Answer from the drawing. Dimensions are ordinates in mm from the lowest x, y and z of the part. A direction names the side the tool comes from. Round coordinates to 2 decimals unless told otherwise and drop trailing zeros. Loops run counter-clockwise (first coordinate to the right, second up) from the corner with the lowest first, then second, coordinate; pieces in that order, holes last. Notation, with made-up numbers: (75.25, -32) - (97.25, -32) arc R21 ccw to (97.25, -12) - close; hole circle Ø11 at (89, 28). An arc over 180 degrees is marked (long way). Answer as CSV lines item,"result". Start each with the question number.
Q1. Section B-B on x = 8 is taken. Write down the section's boundary in (y, z).
Q2. Section C-C on y = 36 is taken. Write down the section's boundary in (x, z), then the cut area to 3 significant figures.
Q3. For the marked faces 4, 5 and 6, determine the directions among +Z, -Z, +X, -X, +Y, -Y from which every point of the face is accessible in a straight line to the end or side of a thin tool.
Q4. Each of these flat-tipped pins is pushed along its axis until it touches: pin 1 Ø11 at (x, z) = (10, 34.5) entering from +Y; pin 2 Ø8 at (y, z) = (36, 25) entering from -X; pin 3 Ø12 at (y, z) = (28, 21) entering from -X; pin 4 Ø12 at (y, z) = (33.5, 30) entering from +X. Where does it stop, or does it pass through?
Q5. Section A-A on y = 30 is taken. Write down the section's boundary in (x, z), then the cut area to 3 significant figures.
Q6. Section D-D on z = 8 is taken. Write down the section's boundary in (x, y).
Q7. Straight lines are drawn through the part: L1, parallel to X at y = 2.2, z = 44; L2, parallel to Z at x = 8, y = 2; L3, parallel to X at y = 16, z = 16. For each, find the intervals that lie inside material, in ascending order. Write a range as [from, to].
Q8. The mould has two halves that part along X. Classify the marked faces 1, 2 and 3: +X half, -X half, draft (parallel to the pull), parting line (faces both ways), or undercut.
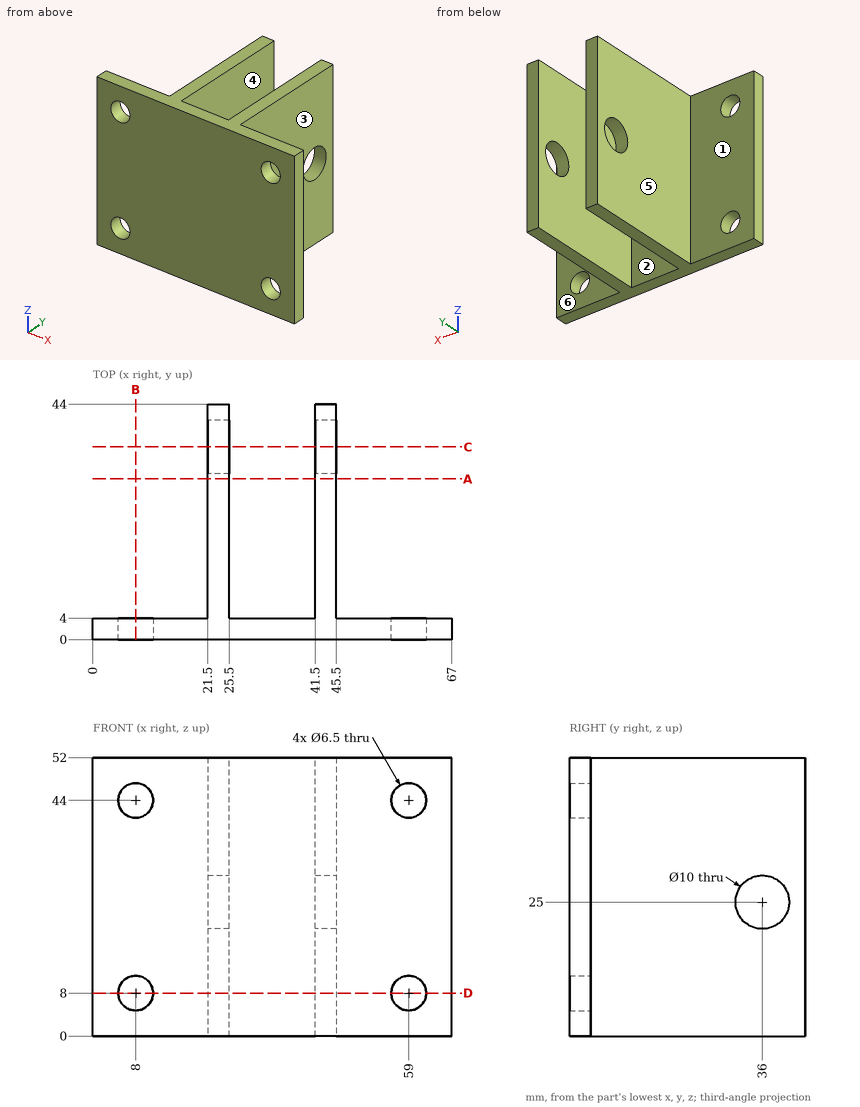
Findings:
1,outline,"(0, 0) - (4, 0) - (4, 4.75) - (0, 4.75) - close; (0, 11.25) - (4, 11.25) - (4, 40.75) - (0, 40.75) - close; (0, 47.25) - (4, 47.25) - (4, 52) - (0, 52) - close"
2,outline,"(21.5, 0) - (25.5, 0) - (25.5, 20) - (21.5, 20) - close; (21.5, 30) - (25.5, 30) - (25.5, 52) - (21.5, 52) - close; (41.5, 0) - (45.5, 0) - (45.5, 20) - (41.5, 20) - close; (41.5, 30) - (45.5, 30) - (45.5, 52) - (41.5, 52) - close"
2,area,"336 mm^2"
3,face 4,"+Z, -Z, +Y"
3,face 5,"+Z, -Z, -X, +Y"
3,face 6,"+Z, -Z, +X, +Y"
4,pin 1,"stops at y = 4"
4,pin 2,"passes through"
4,pin 3,"stops at x = 21.5"
4,pin 4,"stops at x = 45.5"
5,outline,"(21.5, 0) - (25.5, 0) - (25.5, 52) - (21.5, 52) - close; (41.5, 0) - (45.5, 0) - (45.5, 52) - (41.5, 52) - close"
5,area,"416 mm^2"
6,outline,"(0, 0) - (4.75, 0) - (4.75, 4) - (0, 4) - close; (11.25, 0) - (55.75, 0) - (55.75, 4) - (45.5, 4) - (45.5, 44) - (41.5, 44) - (41.5, 4) - (25.5, 4) - (25.5, 44) - (21.5, 44) - (21.5, 4) - (11.25, 4) - close; (62.25, 0) - (67, 0) - (67, 4) - (62.25, 4) - close"
7,L1,"x = [0, 4.75], [11.25, 55.75], [62.25, 67]"
7,L2,"z = [0, 4.75], [11.25, 40.75], [47.25, 52]"
7,L3,"x = [21.5, 25.5], [41.5, 45.5]"
8,face 1,"draft"
8,face 2,"undercut"
8,face 3,"+X half"
